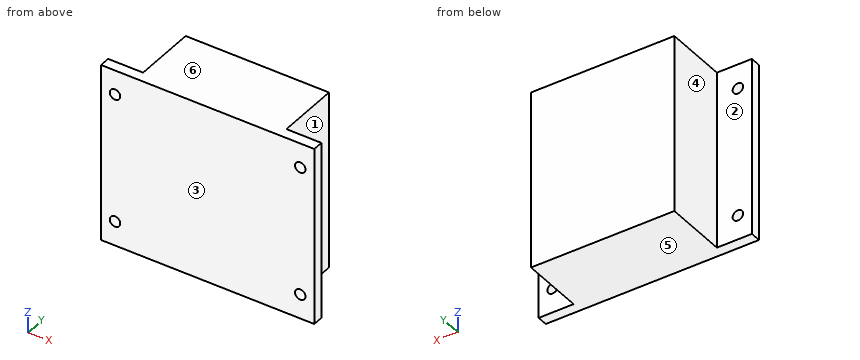
```python
from build123d import *

# Parameters (mm, degrees)
ESBO_O1_W                = 61
ESBO_O1_H                = 51
ESBO_O1_R                = 1.5
RESSALTO_EXTRUS_O1_DEPTH = 21
ESBO_O2_W                = 10
ESBO_O2_H                = 51
CORTE_EXTRUS_O1_DEPTH    = 18


with BuildPart() as part:
    # Esboço1 → Ressalto-extrusão1 (new body)
    with BuildSketch(Plane(origin=(0, 0, 0), x_dir=(1, 0, 0), z_dir=(0, 1, 0))):
        Rectangle(ESBO_O1_W, ESBO_O1_H)
        with Locations(Location((-26.5, 18.5, 0), (0, 0, 90))):
            Circle(ESBO_O1_R, mode=Mode.SUBTRACT)
        with Locations(Location((-26.5, -18.5, 0), (0, 0, 90))):
            Circle(ESBO_O1_R, mode=Mode.SUBTRACT)
        with Locations(Location((26.5, -18.5, 0), (0, 0, 90))):
            Circle(ESBO_O1_R, mode=Mode.SUBTRACT)
        with Locations(Location((26.5, 18.5, 0), (0, 0, 90))):
            Circle(ESBO_O1_R, mode=Mode.SUBTRACT)
    extrude(amount=RESSALTO_EXTRUS_O1_DEPTH)

    # Esboço2 → Corte-extrusão1 (cut)
    with BuildSketch(Plane(origin=(0, 21, 0), x_dir=(1, 0, 0), z_dir=(0, 1, 0))):
        with Locations((-25.5, 0)):
            Rectangle(ESBO_O2_W, ESBO_O2_H)
        with Locations((25.5, 0)):
            Rectangle(ESBO_O2_W, ESBO_O2_H)
    extrude(amount=-CORTE_EXTRUS_O1_DEPTH, mode=Mode.SUBTRACT)


solid = part.part
```
Check sheet for the modelled part. Datum: model origin and axes. Units: mm. Face numbers are marked on the shaded views. A direction names the side the tool comes from. Round coordinates to 2 decimals unless told otherwise and drop trailing zeros. Write each loop counter-clockwise with the first axis right and the second up, starting at its lowest first coordinate (ties: lowest second). Pieces come first, ordered by that corner, then holes. Notation, with made-up numbers: (43.5, 71) -> (91.5, 71) arc R11 cw to (91.5, 89) -> close; hole circle Ø3 at (28, 13). An arc over 180 degrees is marked (long way). One line per question, with ' | ' between items. Start each with the question number.
1. Depth check by flat-ended pin: pin 1 (5 mm diameter, centred on x = 27.5, z = 1.5, fed in from +Y); pin 2 (12 mm diameter, centred on y = 17, z = -14, fed in from -X); pin 3 (5 mm diameter, centred on y = 14.5, z = -9, fed in from +X); pin 4 (2.5 mm diameter, centred on x = -26.5, z = 18.5, fed in from -Y). Enter the tip coordinate at first touch or a pass-through.
2. Release check for a two-part mould opening along Z. For the marked faces 4, 5 and 6 record: +Z half, -Z half, draft (parallel to the pull), parting line (faces both ways), or undercut.
3. Sectioned sample at A-A, the plane x = 26.5. Record the cut outline in (y, z).
4. Sectioned sample at C-C, the plane y = 4. Record the cut outline in (x, z).
5. Scan lines: line 1 along Z through (x, y) = (26.5, 1.4); line 2 along X through (y, z) = (0.7, -18.5); line 3 along X through (y, z) = (17, 10). Record each from-to range of solid material in increasing order. Write a range as from..to.
6. Set-up check for the marked faces 1, 2 and 3: record each of +Z, -Z, +X, -X, +Y, -Y from which the full face is reachable in a straight line by a thin tool's end or side.
7. Sectioned sample at B-B, the plane z = -18.5. Record the cut outline in (x, y).
Taken from the geometry:
1) pin 1: stops at y = 3 | pin 2: stops at x = -20.5 | pin 3: stops at x = 20.5 | pin 4: passes through
2) face 4: draft | face 5: -Z half | face 6: +Z half
3) outline: (0, -25.5) -> (3, -25.5) -> (3, -20) -> (0, -20) -> close; (0, -17) -> (3, -17) -> (3, 17) -> (0, 17) -> close; (0, 20) -> (3, 20) -> (3, 25.5) -> (0, 25.5) -> close
4) outline: (-20.5, -25.5) -> (20.5, -25.5) -> (20.5, 25.5) -> (-20.5, 25.5) -> close
5) line 1: z = -25.5..-20, -17..17, 20..25.5 | line 2: x = -30.5..-28, -25..25, 28..30.5 | line 3: x = -20.5..20.5
6) face 1: +Z, -Z, +X, +Y | face 2: +Z, -Z, -X, +Y | face 3: +Z, -Z, +X, -X, -Y
7) outline: (-30.5, 0) -> (-28, 0) -> (-28, 3) -> (-30.5, 3) -> close; (-25, 0) -> (25, 0) -> (25, 3) -> (20.5, 3) -> (20.5, 21) -> (-20.5, 21) -> (-20.5, 3) -> (-25, 3) -> close; (28, 0) -> (30.5, 0) -> (30.5, 3) -> (28, 3) -> close
